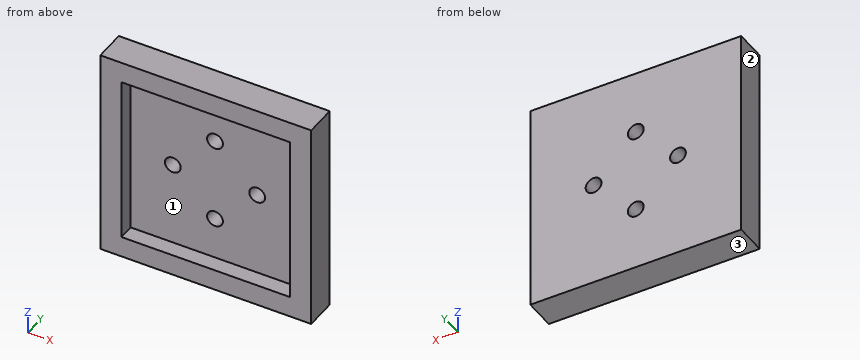
```python
from build123d import *

# Parameters (mm, degrees)
SKETCH1_W           = 40
SKETCH1_H           = 40
SKETCH1_R           = 1.5
BOSS_EXTRUDE1_DEPTH = 3
SKETCH2_W           = 40
SKETCH2_H           = 40
SKETCH2_W_2         = 32
SKETCH2_H_2         = 32
BOSS_EXTRUDE2_DEPTH = 3


with BuildPart() as part:
    # Sketch1 → Boss-Extrude1 (new body)
    with BuildSketch(Plane(origin=(0, 0, 0), x_dir=(1, 0, 0), z_dir=(0, 1, 0))):
        Rectangle(SKETCH1_W, SKETCH1_H)
        with Locations((0, 8)):
            Circle(SKETCH1_R, mode=Mode.SUBTRACT)
        with Locations((8, 0)):
            Circle(SKETCH1_R, mode=Mode.SUBTRACT)
        with Locations((0, -8)):
            Circle(SKETCH1_R, mode=Mode.SUBTRACT)
        with Locations((-8, 0)):
            Circle(SKETCH1_R, mode=Mode.SUBTRACT)
    extrude(amount=BOSS_EXTRUDE1_DEPTH)

    # Sketch2 → Boss-Extrude2 (add)
    with BuildSketch(Plane.XZ):
        Rectangle(SKETCH2_W, SKETCH2_H)
        Rectangle(SKETCH2_W_2, SKETCH2_H_2, mode=Mode.SUBTRACT)
    extrude(amount=BOSS_EXTRUDE2_DEPTH)


solid = part.part
```
Geometry: final body of the model. Coordinates: model frame, mm. Face numbers are marked on the shaded views. Give positions to 0.01 mm unless a question says otherwise; leave off trailing zeros. Order: outer loops, then holes, each group sorted by start corner. A loop starts at its lowest first (then second) coordinate and runs counter-clockwise, first axis right, second up. Notation, with made-up numbers: M 12,-33.75 L 58,-33.75 A15 cw 58,-12.75 Z; hole C -13,-11.75 d11. An arc over 180 degrees is marked long. Answer as CSV lines item,"result". Start each with the question number.
1) Cut plane B-B (y = 0.6). Output: boundary loops of the cut face in (x, z), then the cut area to 3 significant figures.
2) Cut plane D-D (z = 8). Output: boundary loops of the cut face in (x, y).
3) Cut plane C-C (z = 0). Output: boundary loops of the cut face in (x, y).
4) Line query: line 1 (Z direction, x = 0, y = 1.4); line 2 (X direction, y = 2.1, z = 8). Output: solid intervals per line, ascending. Write a range as from..to.
5) Mould query, pull axis Z, two halves, no side actions, for the marked faces 1, 2 and 3. Classes: +Z half, -Z half, draft (parallel to the pull), parting line (faces both ways), or undercut.
6) First-contact query: P1, Ø2.5, axis at x = 8, z = 0, coming from the +Y side. Flat tip, straight axial feed; report the tip coordinate or a pass-through.
7) Cut plane A-A (x = 8). Output: boundary loops of the cut face in (y, z), then the cut area to 3 significant figures.
Findings below:
1,outline,"M -20,-20 L 20,-20 L 20,20 L -20,20 Z; hole C -8,0 d3; hole C 0,-8 d3; hole C 0,8 d3; hole C 8,0 d3"
1,area,"1,570 mm²"
2,outline,"M -20,-3 L -16,-3 L -16,0 L -1.5,0 L -1.5,3 L -20,3 Z; M 1.5,0 L 16,0 L 16,-3 L 20,-3 L 20,3 L 1.5,3 Z"
3,outline,"M -20,-3 L -16,-3 L -16,0 L -9.5,0 L -9.5,3 L -20,3 Z; M -6.5,0 L 6.5,0 L 6.5,3 L -6.5,3 Z; M 9.5,0 L 16,0 L 16,-3 L 20,-3 L 20,3 L 9.5,3 Z"
4,line 1,"z = -20..-9.5, -6.5..6.5, 9.5..20"
4,line 2,"x = -20..-1.5, 1.5..20"
5,face 1,"undercut"
5,face 2,"draft"
5,face 3,"-Z half"
6,P1,"passes through"
7,outline,"M -3,-20 L 3,-20 L 3,-1.5 L 0,-1.5 L 0,-16 L -3,-16 Z; M -3,16 L 0,16 L 0,1.5 L 3,1.5 L 3,20 L -3,20 Z"
7,area,"135 mm²"
